Autodesk Inventor part; units mm, degrees
ref_plane "YZ Plane" through (0, 0, 0) normal (1, 0, 0) x (0, 1, 0)
ref_plane "XZ Plane" through (0, 0, 0) normal (0, 1, 0) x (-1, 0, 0)
ref_plane "XY Plane" through (0, 0, 0) normal (0, 0, 1) x (1, 0, 0)
sketch "Sketch1" plane through (0, 0, 0) normal (1, 0, 0) x (0, 1, 0)
  line L0 (0, 0) -> (0, -100)
  line L1 (0, 0) -> (8, 0)
  line L2 (8, 0) -> (8, -20)
  line L3 (8, -20) -> (15, -20)
  line L4 (15, -20) -> (15, -50)
  line L5 (15, -50) -> (22.5, -50)
  line L6 (22.5, -50) -> (22.5, -65)
  line L7 (22.5, -65) -> (10, -65)
  line L8 (10, -65) -> (10, -100)
  line L9 (10, -100) -> (0, -100)
  dimension "d0" = 100
  dimension "d1" = 8
  dimension "d2" = 20
  dimension "d3" = 7
  dimension "d4" = 30
  dimension "d5" = 7.5
  dimension "d6" = 15
  dimension "d7" = 12.5
revolve "Revolution1" add sketch "Sketch1" angle 360 about axis through (0, 0, 0) along (0, 0, -1)
chamfer "Chamfer1" distance 2 angle 45 1 edges at (0, -15, -20)
chamfer "Chamfer2" distance 1 angle 45 1 edges at (0, -8, 0)
fillet "Fillet1" radius 2 1 edges at (0, -22.5, -50)
fillet "Fillet2" radius 2 1 edges at (0, -22.5, -65)
fillet "Fillet3" radius 4 1 edges at (0, -10, -65)
chamfer "Chamfer3" distance 1.5 angle 45 1 edges at (0, -10, -100)
The listing builds one solid part. Answer for the finished solid, in the listing's coordinates (mm). A direction names the side the tool comes from. Give positions to 0.01 mm unless a question says otherwise; leave off trailing zeros. Loops run counter-clockwise (first coordinate to the right, second up) from the corner with the lowest first, then second, coordinate; pieces in that order, holes last. Notation, with made-up numbers: (40, -5) - (66, -5) arc R29 cw to (66, 23) - close; hole circle Ø6 at (16.5, 78). An arc over 180 degrees is marked (long way). Answer as a JSON object with one key per item and string values.
1. Flat-ended cylindrical pins translate along their axes: pin 1 Ø2 at (x, z) = (12, -24.5) entering from +Y; pin 2 Ø8 at (y, z) = (-17.5, -18) entering from +X; pin 3 Ø13 at (x, y) = (6, -5.5) entering from +Z; pin 4 Ø10 at (x, z) = (13, -60.5) entering from +Y. Find the tip coordinate at first contact, or state that the pin passes through.
Determined:
{"pin 1": "y = 10.2", "pin 2": "through", "pin 3": "z = 0", "pin 4": "y = 21.03"}
2. A cutting plane is placed at C-C (z = -75). Write down the section's boundary in (x, y).
Determined:
{"outline": "circle Ø20 at (0, 0)"}
3. Find the intervals of material crossed by L1, parallel to Z at x = 18.5, y = 5; L2, parallel to X at y = 0, z = -81.5; L3, parallel to X at y = 6, z = -91, in increasing order. Write a range as [from, to].
Determined:
{"L1": "[-65, -50]", "L2": "[-10, 10]", "L3": "[-8, 8]"}
4. A cutting plane is placed at D-D (z = -37.5). Write down the section's boundary in (x, y), then the cut area to 3 significant figures.
Determined:
{"outline": "circle Ø30 at (0, 0)", "area": "707 mm²"}
5. A cutting plane is placed at A-A (x = 0). Write down the section's boundary in (y, z).
Determined:
{"outline": "(-22.5, -63) arc R2 ccw to (-20.5, -65) - (-14, -65) arc R4 cw to (-10, -69) - (-10, -98.5) - (-8.5, -100) - (8.5, -100) - (10, -98.5) - (10, -69) arc R4 cw to (14, -65) - (20.5, -65) arc R2 ccw to (22.5, -63) - (22.5, -52) arc R2 ccw to (20.5, -50) - (15, -50) - (15, -22) - (13, -20) - (8, -20) - (8, -1) - (7, 0) - (-7, 0) - (-8, -1) - (-8, -20) - (-13, -20) - (-15, -22) - (-15, -50) - (-20.5, -50) arc R2 ccw to (-22.5, -52) - close"}
6. For faces 1 (the flat face through (0, 0, 0)), 2 (the cylindrical face through (-9.76, -2.17, -83.96)), 3 (the flat face through (-15.1, 1.4, -50)), determine the directions among +Z, -Z, +X, -X, +Y, -Y from which every point of the face is accessible in a straight line to the end or side of a thin tool.
Determined:
{"face 1": "+Z, +X, -X, +Y, -Y", "face 2": "-Z", "face 3": "+Z"}
